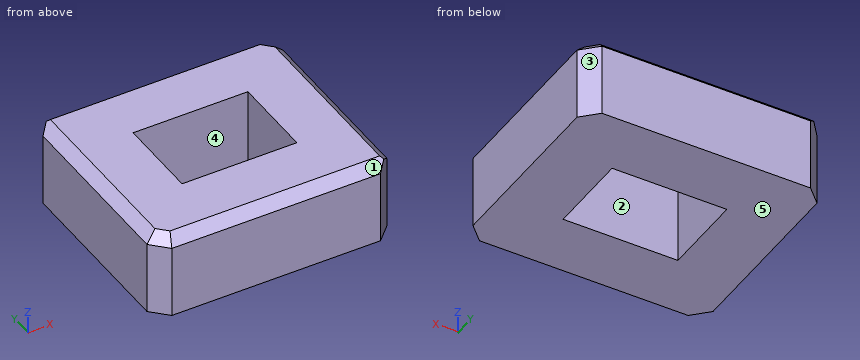
```python
from build123d import *

# Parameters (mm, degrees)
SALIENTE_EXTRUIR1_DEPTH = 8
CROQUIS2_W              = 11
CROQUIS2_H              = 8
CORTAR_EXTRUIR1_DEPTH   = 18.211914478
CHAFL_N1_SIZE           = 1


with BuildPart() as part:
    # Croquis1 → Saliente-Extruir1 (new body)
    with BuildSketch(Plane.XY):
        Polygon((-11.5, 8.5), (-10, 10), (10, 10), (11.5, 8.5), (11.5, -8.5), (10, -10), (-10, -10), (-11.5, -8.5), align=None)
    extrude(amount=SALIENTE_EXTRUIR1_DEPTH)

    # Croquis2 → Cortar-Extruir1 (cut, through all)
    with BuildSketch(Plane.XY.offset(8)):
        Rectangle(CROQUIS2_W, CROQUIS2_H)
    extrude(amount=-CORTAR_EXTRUIR1_DEPTH, mode=Mode.SUBTRACT)

    # Chaflán1
    # the kernel refuses this chamfer: 1 mm, written as the material it takes off along each edge
    with BuildSketch(Plane(origin=(-11.5, -11.071682988, 8), x_dir=(-0.027495876610585623, 0, -0.9996219169112968), z_dir=(0, 1, 0))) as chafl_n1_piece_1:
        Polygon((CHAFL_N1_SIZE * 0.999621916911, -CHAFL_N1_SIZE * 0.0274958766106), (-CHAFL_N1_SIZE * 0.0274958766106, -CHAFL_N1_SIZE * 0.999621916911), (0, 0), align=None)
    extrude(amount=22.143365976, mode=Mode.SUBTRACT)
    with BuildSketch(Plane(origin=(-8.18154552, -11.81845448, 8), x_dir=(0.7068394360706735, 0.7068394360706735, 0.02749587661058563), z_dir=(-0.7071067811865476, 0.7071067811865476, 0)), Plane(origin=(8.18154552, 11.81845448, 8), x_dir=(-0.7068394360706735, -0.7068394360706735, 0.02749587661058563), z_dir=(0.7071067811865476, -0.7071067811865476, 0))) as chafl_n1_piece_2:
        Polygon((CHAFL_N1_SIZE * 0.999621916911, CHAFL_N1_SIZE * 0.0274958766106), (-CHAFL_N1_SIZE * 0.0274958766106, CHAFL_N1_SIZE * 0.999621916911), (0, 0), align=None)
    extrude(amount=7.264686319, mode=Mode.SUBTRACT)
    with BuildSketch(Plane(origin=(12.571682988, -10, 8), x_dir=(0, 0.9996219169112968, 0.027495876610585647), z_dir=(-1, 0, 0))) as chafl_n1_piece_3:
        Polygon((CHAFL_N1_SIZE * 0.999621916911, CHAFL_N1_SIZE * 0.0274958766106), (-CHAFL_N1_SIZE * 0.0274958766106, CHAFL_N1_SIZE * 0.999621916911), (0, 0), align=None)
    extrude(amount=25.143365976, mode=Mode.SUBTRACT)
    with BuildSketch(Plane(origin=(11.5, 11.071682988, 8), x_dir=(-0.9996219169112968, 0, 0.027495876610585647), z_dir=(0, -1, 0))) as chafl_n1_piece_4:
        Polygon((CHAFL_N1_SIZE * 0.999621916911, CHAFL_N1_SIZE * 0.0274958766106), (-CHAFL_N1_SIZE * 0.0274958766106, CHAFL_N1_SIZE * 0.999621916911), (0, 0), align=None)
    extrude(amount=22.143365976, mode=Mode.SUBTRACT)
    with BuildSketch(Plane(origin=(-12.571682988, 10, 8), x_dir=(0, 0.027495876610585623, -0.9996219169112968), z_dir=(1, 0, 0))) as chafl_n1_piece_5:
        Polygon((CHAFL_N1_SIZE * 0.999621916911, -CHAFL_N1_SIZE * 0.0274958766106), (-CHAFL_N1_SIZE * 0.0274958766106, -CHAFL_N1_SIZE * 0.999621916911), (0, 0), align=None)
    extrude(amount=25.143365976, mode=Mode.SUBTRACT)


solid = part.part
```
CAD build for the part. Positions are in the model's coordinates, mm. Face numbers are marked on the shaded views. A direction names the side the tool comes from. Coordinates: 2 decimals unless noted, no trailing zeros. Order: outer loops, then holes, each group sorted by start corner. A loop starts at its lowest first (then second) coordinate and runs counter-clockwise, first axis right, second up.
(1) Which spindle directions (+Z, -Z, +X, -X, +Y, -Y) get a long thin tool onto all of the face, cutting with end or side? Do the marked faces 4 and 5. Say none if no direction does.
Solution:
face 4: +Z, -Z
face 5: -Z, +X, -X, +Y, -Y
(2) Saw through at B-B, the plane z = 5.5. Write the cut outline in (x, y).
Solution:
outline: (-11.5, -8.5) - (-10, -10) - (10, -10) - (11.5, -8.5) - (11.5, 8.5) - (10, 10) - (-10, 10) - (-11.5, 8.5) - close; hole (-5.5, -4) - (5.5, -4) - (5.5, 4) - (-5.5, 4) - close
(3) Saw through at C-C, the plane x = 3.5. Write the cut outline in (y, z).
Solution:
outline: (-10, 0) - (-4, 0) - (-4, 8) - (-9, 8) - (-10, 7) - close; (4, 0) - (10, 0) - (10, 7) - (9, 8) - (4, 8) - close
(4) Drill centre lines: L1, parallel to X at y = 3.75, z = 0.75; L2, parallel to Y at x = 4.25, z = 6; L3, parallel to Y at x = 10.75, z = 5. Where is each one in solid material? Low to high.
Solution:
L1: x = -11.5 to -5.5, 5.5 to 11.5
L2: y = -10 to -4, 4 to 10
L3: y = -9.25 to 9.25
(5) Mould opens along X. For the marked faces 1, 2 and 3 say: released by +X, released by -X, zero draft, split by the parting line, or undercut.
Solution:
face 1: zero draft
face 2: undercut
face 3: released by +X
(6) Saw through at A-A, the plane y = -3. Write the cut outline in (x, z), and give its area (3 significant figures).
Solution:
outline: (-11.5, 0) - (-5.5, 0) - (-5.5, 8) - (-10.5, 8) - (-11.5, 7) - close; (5.5, 0) - (11.5, 0) - (11.5, 7) - (10.5, 8) - (5.5, 8) - close
area: 95.0 mm2
